The listing builds one solid part. Answer for the finished solid, in the listing's coordinates (mm). Coordinates: 2 decimals unless noted, no trailing zeros. Order: outer loops, then holes, each group sorted by start corner. A loop starts at its lowest first (then second) coordinate and runs counter-clockwise, first axis right, second up. Notation, with made-up numbers: (56, 23.25) - (108, 23.25) arc R23 ccw to (108, 47.25) - close; hole circle Ø5 at (22, 1). An arc over 180 degrees is marked (long way). Use a Markdown table: item, result. Add a question column.
Item 1: The part is cut by section B-B, the plane y = 3.75. Give the vertices of the cut face in (x, z), then the cut area to 3 significant figures.
Item 2: The part is cut by section C-C, the plane x = -20. Give the vertices of the cut face in (y, z), then the cut area to 3 significant figures.
Item 3: The part is cut by section A-A, the plane x = -152.4. Give the vertices of the cut face in (y, z), then the cut area to 3 significant figures.
Item 4: The part is cut by section D-D, the plane x = 140.5. Give the vertices of the cut face in (y, z).
Item 5: Find the intervals of material crossed by line 1 along X through (y, z) = (3.75, 749.3); line 2 along Z through (x, y) = (52.5, 2); line 3 along Z through (x, y) = (-160.5, 5.25), in increasing order.
from build123d import *

# Parameters (mm, degrees)
SKETCH1_W           = 482.6
SKETCH1_H           = 1651
BOSS_EXTRUDE1_DEPTH = 6.35
SKETCH2_R           = 43.923649364
CUT_EXTRUDE1_DEPTH  = 861.067591821
CUT_EXTRUDE3_DEPTH  = 861.067591821


with BuildPart() as part:
    # Sketch1 → Boss-Extrude1 (new body)
    with BuildSketch(Plane(origin=(0, 0, 0), x_dir=(1, 0, 0), z_dir=(0, 1, 0))):
        Rectangle(SKETCH1_W, SKETCH1_H)
    extrude(amount=BOSS_EXTRUDE1_DEPTH)

    # Sketch2 → Cut-Extrude1 (cut, through all)
    with BuildSketch(Plane(origin=(0, 6.35, 0), x_dir=(1, 0, 0), z_dir=(0, 1, 0))):
        with Locations(Location((-152.4, -749.3, 0), (0, 0, 270))):
            Circle(SKETCH2_R)
    extrude(amount=-CUT_EXTRUDE1_DEPTH, mode=Mode.SUBTRACT)

    # Sketch4 → Cut-Extrude3 (cut, through all)
    with BuildSketch(Plane.XZ):
        with BuildLine():
            Line((-50.444519558, 744.293611593), (-50.444519558, 825.5))
            Line((-50.444519558, 825.5), (13.055480442, 825.5))
            Line((13.055480442, 825.5), (13.055480442, 744.293611593))
            ThreePointArc((13.055480442, 744.293611593), (-18.694519558, 712.543611593), (-50.444519558, 744.293611593))
        make_face()
        with BuildLine():
            Line((25.755480442, 744.293611593), (25.755480442, 825.5))
            Line((25.755480442, 825.5), (89.255480442, 825.5))
            Line((89.255480442, 825.5), (89.255480442, 744.293611593))
            ThreePointArc((89.255480442, 744.293611593), (57.505480442, 712.543611593), (25.755480442, 744.293611593))
        make_face()
        with BuildLine():
            Line((101.955480442, 744.293611593), (101.955480442, 825.5))
            Line((101.955480442, 825.5), (165.455480442, 825.5))
            Line((165.455480442, 825.5), (165.455480442, 744.293611593))
            ThreePointArc((165.455480442, 744.293611593), (133.705480442, 712.543611593), (101.955480442, 744.293611593))
        make_face()
    extrude(amount=-CUT_EXTRUDE3_DEPTH, mode=Mode.SUBTRACT)


solid = part.part
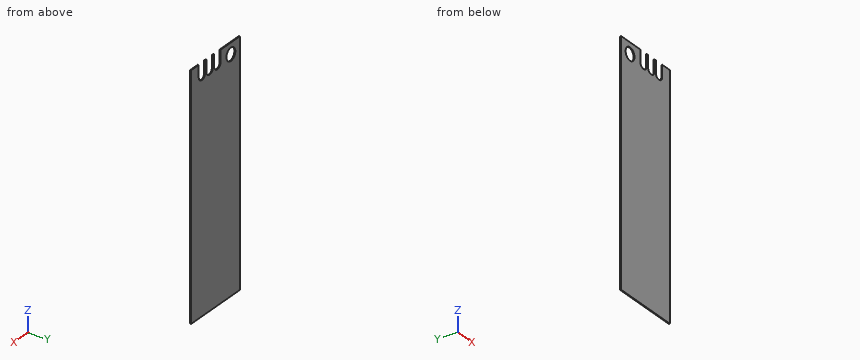
Solution:
| question | item | result |
|---|---|---|
| 1 | outline | (-241.3, -825.5) - (241.3, -825.5) - (241.3, 825.5) - (165.46, 825.5) - (165.46, 744.29) arc R31.75 cw to (101.96, 744.29) - (101.96, 825.5) - (89.26, 825.5) - (89.26, 744.29) arc R31.75 cw to (25.76, 744.29) - (25.76, 825.5) - (13.06, 825.5) - (13.06, 744.29) arc R31.75 cw to (-50.44, 744.29) - (-50.44, 825.5) - (-241.3, 825.5) - close; hole circle Ø87.85 at (-152.4, 749.3) |
| 1 | area | 770,000 mm2 |
| 2 | outline | (0, -825.5) - (6.35, -825.5) - (6.35, 712.57) - (0, 712.57) - close |
| 2 | area | 9,770 mm2 |
| 3 | outline | (0, -825.5) - (6.35, -825.5) - (6.35, 705.38) - (0, 705.38) - close; (0, 793.22) - (6.35, 793.22) - (6.35, 825.5) - (0, 825.5) - close |
| 3 | area | 9,930 mm2 |
| 4 | outline | (0, -825.5) - (6.35, -825.5) - (6.35, 713.28) - (0, 713.28) - close |
| 5 | line 1 | x = -241.3 to -196.32, -108.48 to -50.44, 13.06 to 25.76, 89.26 to 101.96, 165.46 to 241.3 |
| 5 | line 2 | z = -825.5 to 712.94 |
| 5 | line 3 | z = -825.5 to 706.13, 792.47 to 825.5 |
